from build123d import *

# Parameters (mm, degrees)
CROQUIS1_R              = 49
CROQUIS1_R_2            = 4
CROQUIS1_R_3            = 1.5
SALIENTE_EXTRUIR1_DEPTH = 2.5
CROQUIS2_R              = 11
CORTAR_EXTRUIR1_DEPTH   = 0.5
REDONDEO1_R             = 2
REDONDEO2_R             = 2
REDONDEO3_R             = 5


with BuildPart() as part:
    # Croquis1 → Saliente-Extruir1 (new body)
    with BuildSketch(Plane(origin=(0, 0, 0), x_dir=(1, 0, 0), z_dir=(0, 1, 0))):
        with Locations(Location((0, 0, 0), (0, 0, 270))):
            Circle(CROQUIS1_R)
        with Locations(Location((0, 0, 0), (0, 0, 270))):
            Circle(CROQUIS1_R_2, mode=Mode.SUBTRACT)
        with Locations(Location((7.25, 0, 0), (0, 0, 270))):
            Circle(CROQUIS1_R_3, mode=Mode.SUBTRACT)
        with Locations(Location((-7.25, 0, 0), (0, 0, 90))):
            Circle(CROQUIS1_R_3, mode=Mode.SUBTRACT)
    extrude(amount=SALIENTE_EXTRUIR1_DEPTH)

    # Croquis2 → Cortar-Extruir1 (cut)
    with BuildSketch(Plane(origin=(0, 2.5, 0), x_dir=(1, 0, 0), z_dir=(0, 1, 0))):
        with Locations(Location((0, 0, 0), (0, 0, 270))):
            Circle(CROQUIS2_R)
    extrude(amount=-CORTAR_EXTRUIR1_DEPTH, mode=Mode.SUBTRACT)

    # Redondeo1
    # the kernel refuses this fillet: 2 mm, written as the material it adds along each edge
    with BuildSketch(Plane(origin=(0, 2, 0), x_dir=(0, 0, 1), z_dir=(-1, 0, 0))) as redondeo1_piece_1:
        with BuildLine():
            CenterArc((9.677124344, 2), REDONDEO1_R, 270, 41.409622109)
            Line((9.677124344, 0), (9.677124344, -0.04))
            Line((9.677124344, -0.04), (11, -0.04))
            Line((11, -0.04), (11.04, 0))
            ThreePointArc((11.04, 0), (11.04, 0.25), (11.026457513, 0.47))
            Line((11.026457513, 0.47), (11, 0.5))
        make_face()
    revolve(axis=Axis((0, 2, 0), (0, 1, 0)))

    # Redondeo2
    redondeo2_edges = [part.edges().sort_by_distance(p)[0] for p in [
        (0, 2.5, -11),
    ]]
    fillet(redondeo2_edges, radius=REDONDEO2_R)

    # Redondeo3
    # the kernel refuses this fillet: 5 mm, written as the material it takes off along each edge
    with BuildSketch(Plane(origin=(0, 2.5, 0), x_dir=(0, 0, 1), z_dir=(-1, 0, 0))) as redondeo3_piece_1:
        with BuildLine():
            CenterArc((44.669872981, -5), REDONDEO3_R, 30, 60)
            Line((49, -2.5), (49.08660254, -2.45))
            ThreePointArc((49.08660254, -2.45), (49.1, -1.25), (49.1, 0))
            Line((49.1, 0), (49, 0.1))
            Line((49, 0.1), (44.669872981, 0.1))
            Line((44.669872981, 0.1), (44.669872981, 0))
        make_face()
    revolve(axis=Axis((0, 2.5, 0), (0, 1, 0)), mode=Mode.SUBTRACT)


solid = part.part
Part model, mm, in its own coordinate system. A direction names the side the tool comes from. Give positions to 0.01 mm unless a question says otherwise; leave off trailing zeros. Write each loop counter-clockwise with the first axis right and the second up, starting at its lowest first coordinate (ties: lowest second). Pieces come first, ordered by that corner, then holes.
1) Pin check, flat tips, straight feed: pin 1 (15.5 mm diameter, centred on x = -0.5, z = 0, fed in from +Y); pin 2 (1 mm diameter, centred on x = 7, y = 2, fed in from +Z); pin 3 (1.5 mm diameter, centred on x = -15.5, y = 1, fed in from +Z); pin 4 (5 mm diameter, centred on x = 32, z = 28.5, fed in from -Y). Stop position of each tip, or through.
Resolved:
pin 1: stops at y = 2
pin 2: stops at z = 47.16
pin 3: stops at z = 46.38
pin 4: stops at y = 0
2) Cut at A-A on z = 0. State how many separate pieces and enclosed holes the cut face has, then the cut area to 3 significant figures.
Resolved:
separate pieces: 4
enclosed holes: 0
area: 200 mm2
3) Two-plate mould, pull along Y, no slides. Class faces 3 (the face through (-10, 0, -1)), 4 (the face through (-9, 2.5, 9)), 5 (the face through (-3.905, 0.986, -0.867)): released by +Y, released by -Y, zero draft, split by the parting line, or undercut.
Resolved:
face 3: released by -Y
face 4: released by +Y
face 5: zero draft
4) Probe L1, parallel to X at y = 1.1, z = 0; L2, parallel to X at y = 1.05, z = -18; L3, parallel to X at y = 0.4, z = 1. List the from-to ranges inside material, lowest first.
Resolved:
L1: x = -48.14 to -8.75, -5.75 to -4, 4 to 5.75, 8.75 to 48.14
L2: x = -44.7 to 44.7
L3: x = -48.73 to -8.37, -6.13 to -3.87, 3.87 to 6.13, 8.37 to 48.73
5) Which spindle directions (+Z, -Z, +X, -X, +Y, -Y) get a long thin tool onto all of the face, cutting with end or side? Do faces 1 (the face through (0.1, 2, 4.2)), 2 (the face through (5.786, 0.986, -0.325)). Say none if no direction does.
Resolved:
face 1: +Y
face 2: +Y, -Y
6) Cut at B-B on y = 1.15. Write the cut outline in (x, z).
Resolved:
outline: circle Ø96.17 at (0, 0); hole circle Ø3 at (-7.25, 0); hole circle Ø8 at (0, 0); hole circle Ø3 at (7.25, 0)
